Verification items for the finished model (mm, model axes). Face numbers are marked on the shaded views. A direction names the side the tool comes from. Coordinates: 2 decimals unless noted, no trailing zeros. Write each loop counter-clockwise with the first axis right and the second up, starting at its lowest first coordinate (ties: lowest second). Pieces come first, ordered by that corner, then holes. Notation, with made-up numbers: M 46.5,-36 L 79.5,-36 A18 cw 79.5,-24 Z; hole C 83,77 d9. An arc over 180 degrees is marked long. Answer in a Markdown table with one row per item.
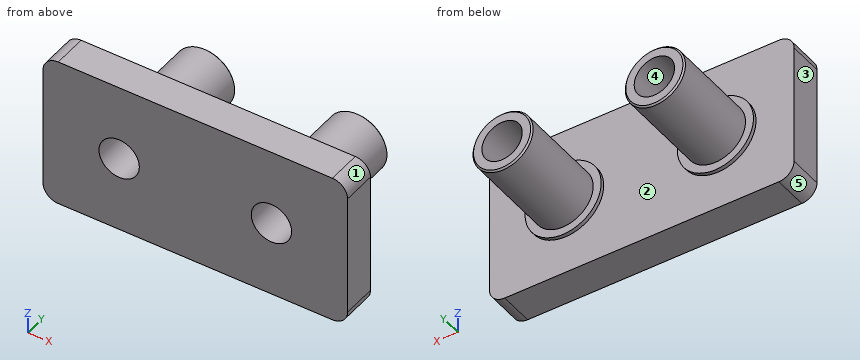
Autodesk Inventor part; units mm, degrees
ref_plane "YZ Plane" through (0, 0, 0) normal (1, 0, 0) x (0, 1, 0)
ref_plane "XZ Plane" through (0, 0, 0) normal (0, 1, 0) x (-1, 0, 0)
ref_plane "XY Plane" through (0, 0, 0) normal (0, 0, 1) x (1, 0, 0)
sketch "スケッチ1" plane through (0, 0, 0) normal (0, 1, 0) x (-1, 0, 0)
  line L0 (20, 10) -> (-20, 10)
  line L1 (-20, 10) -> (-20, -10)
  line L2 (-20, -10) -> (20, -10)
  line L3 (20, -10) -> (20, 10)
  line L4 (20, 10) -> (-20, -10) construction
  line L5 (-20, 10) -> (20, -10) construction
  point P0 (0, 0)
  dimension "d0" = 40
  dimension "d1" = 20
extrude "押し出し1" add sketch "スケッチ1" along normal blind 4.5
sketch "スケッチ2" plane through (0, 4.5, 0) normal (0, 1, 0) x (1, 0, 0)
  circle A0 centre (-10, 0) radius 5
  circle A1 centre (10, 0) radius 5
  point P0 (0, 0)
  dimension "d4" = 10
  dimension "d5" = 10
  dimension "d6" = 10
  dimension "d7" = 10
extrude "押し出し2" add sketch "スケッチ2" along normal blind 0.5
sketch "スケッチ3" plane through (-10, 5, 0) normal (0, 1, 0) x (1, 0, 0)
  circle A0 centre (0, 0) radius 5
  circle A1 centre (20, 0) radius 5
  circle A2 centre (0, 0) radius 3.95
  circle A3 centre (20, 0) radius 3.95
  point P0 (10, 0)
  dimension "d10" = 7.9
  dimension "d11" = 7.9
extrude "押し出し3" add sketch "スケッチ3" along normal blind 12 contours A2 | A3
sketch "スケッチ5" plane through (-10, 17, 0) normal (0, 1, 0) x (1, 0, 0)
  circle A0 centre (0, 0) radius 3.95
  circle A1 centre (20, 0) radius 3.95
  point P0 (10, 0)
hole "穴2" at (10, 17, 0) at (-10, 17, 0) direction (0, -1, 0) diameter 5.3 end through all
chamfer "面取り2" distance 0.2 angle 45 2 edges at (-13.95, 17, 0) (6.05, 17, 0)
fillet "フィレット2" radius 2 4 edges at (20, 2.25, 10) (20, 2.25, -10) (-20, 2.25, 10) (-20, 2.25, -10)
equation "\"d5\" = d4"
equation "\"d11\" = d10"
properties part number "scara-base4" material "ABS プラスチック"
1) Tool access check on the marked faces 1 and 2. Record the directions out of +Z, -Z, +X, -X, +Y, -Y that give a thin tool (end or side, any length) a straight path to the whole face; none if there is none.
Response values:
| item | result |
|---|---|
| face 1 | +Z, +X, +Y, -Y |
| face 2 | +Y |
2) Sectioned sample at D-D (y = 3). Record the cut outline in (x, z), then the cut area to 3 significant figures.
Response values:
| item | result |
|---|---|
| outline | M -20,-8 A2 ccw -18,-10 L 18,-10 A2 ccw 20,-8 L 20,8 A2 ccw 18,10 L -18,10 A2 ccw -20,8 Z; hole C -10,0 d5.3; hole C 10,0 d5.3 |
| area | 752 mm² |
3) Release check for a two-part mould opening along Z. For the marked faces 3, 4 and 5 record: +Z half, -Z half, draft (parallel to the pull), parting line (faces both ways), or undercut.
Response values:
| item | result |
|---|---|
| face 3 | draft |
| face 4 | undercut |
| face 5 | -Z half |
4) Sectioned sample at B-B (z = 0). Give the number of separate pieces and of enclosed holes in the cut face, then the cut area to 3 significant figures.
Response values:
| item | result |
|---|---|
| separate pieces | 3 |
| enclosed holes | 0 |
| area | 199 mm² |
5) Depth check by flat-ended pin: pin 1 (1 mm diameter, centred on y = 9, z = -1, fed in from -X); pin 2 (5 mm diameter, centred on x = -14, z = -2, fed in from +Y); pin 3 (4 mm diameter, centred on y = 8.5, z = -4, fed in from -X); pin 4 (4 mm diameter, centred on y = 11, z = 2.5, fed in from +X). Enter the tip coordinate at first touch or a pass-through.
Response values:
| item | result |
|---|---|
| pin 1 | stops at x = -13.92 |
| pin 2 | stops at y = 17 |
| pin 3 | stops at x = -13.41 |
| pin 4 | stops at x = 13.92 |
6) Sectioned sample at A-A (x = 10). Record the cut outline in (y, z).
Response values:
| item | result |
|---|---|
| outline | M 0,-10 L 4.5,-10 L 4.5,-5 L 5,-5 L 5,-3.95 L 16.8,-3.95 L 17,-3.75 L 17,-2.65 L 0,-2.65 Z; M 0,2.65 L 17,2.65 L 17,3.75 L 16.8,3.95 L 5,3.95 L 5,5 L 4.5,5 L 4.5,10 L 0,10 Z |
7) Thickness scan on L1, parallel to X at y = 4, z = 0; L2, parallel to X at y = 12.5, z = 0; L3, parallel to Z at x = -10, y = 6. Record the ranges inside material, lowest first. Write a range as [from, to].
Response values:
| item | result |
|---|---|
| L1 | x = [-20, -12.65], [-7.35, 7.35], [12.65, 20] |
| L2 | x = [-13.95, -12.65], [-7.35, -6.05], [6.05, 7.35], [12.65, 13.95] |
| L3 | z = [-3.95, -2.65], [2.65, 3.95] |
8) Sectioned sample at C-C (y = 11.25). Record the cut outline in (x, z).
Response values:
| item | result |
|---|---|
| outline | C -10,0 d7.9; C 10,0 d7.9; hole C -10,0 d5.3; hole C 10,0 d5.3 |
